Solid Edge part; units mm, degrees
sketch "Sketch1" plane through (0, 0, 0) normal (0, 0, 1) x (1, 0, 0)
  line L0 (20.5, -19.5) -> (28, -19.5)
  line L1 (28, -19.5) -> (28, -16.5)
  line L2 (28, -16.5) -> (24, -16.5)
  line L3 (24, -16.5) -> (24, 16.5)
  line L4 (24, 16.5) -> (28, 16.5)
  line L5 (28, 16.5) -> (28, 19.5)
  line L6 (28, 19.5) -> (20.5, 19.5)
  line L7 (20.5, -19.5) -> (20.5, 19.5)
revolve "RevolvedProtrusion1" add sketch "Sketch1" angle 180 about axis through (0, 54, 0) along (0, -1, 0)
sketch "Sketch2" plane through (0, 0, 0) normal (0, 0, 1) x (1, 0, 0)
  circle A0 centre (0, 0) radius 1
extrude "ExtrudedCutout_1" cut sketch "Sketch2" along normal mid plane 257.4558
sketch "Sketch3" plane through (0, 0, 0) normal (1, 0, 0) x (0, 1, 0)
  line L0 (-19.5, 0) -> (-19.5, 1.5)
  line L1 (-19.5, 1.5) -> (19.5, 1.5)
  line L2 (19.5, 1.5) -> (19.5, 0)
  line L3 (19.5, 0) -> (-19.5, 0)
extrude "ExtrudedCutout_2" cut sketch "Sketch3" along normal mid plane 153.986
Geometry: final body of the model. Coordinates: model frame, mm. A direction names the side the tool comes from. Give positions to 0.01 mm unless a question says otherwise; leave off trailing zeros. Order: outer loops, then holes, each group sorted by start corner. A loop starts at its lowest first (then second) coordinate and runs counter-clockwise, first axis right, second up. Notation, with made-up numbers: M 49,78 L 75,78 A11 cw 75,91 Z; hole C 58.5,-35.75 d1. An arc over 180 degrees is marked long. Answer as CSV lines item,"result". Start each with the question number.
1) Cut plane B-B (z = 25). Output: boundary loops of the cut face in (x, y).
2) Cut plane D-D (y = 0). Output: boundary loops of the cut face in (x, z).
3) First-contact query: P1, Ø5, axis at y = -1.5, z = 24, coming from the +X side; P2, Ø12, axis at y = 3.5, z = 25, coming from the +X side; P3, Ø3, axis at x = 5.5, y = 0.5, coming from the +Z side. Flat tips, straight axial feed; report the tip coordinate or a pass-through.
4) Set-up query: faces 1 (the flat face through (-2, 16.5, 25)), 2 (the cylindrical face through (-0.43, 4.606, 20.495)). Return all of +Z, -Z, +X, -X, +Y, -Y with unobstructed straight access to the full face (end or side cutting, diameter ignored); none if empty.
5) Line query: line 1 (Y direction, x = -2.5, z = 26); line 2 (Y direction, x = 0, z = 21.8); line 3 (X direction, y = 1.5, z = 10). Output: solid intervals per line, ascending. Write a range as from..to.
6) Mould query, pull axis Y, two halves, no side actions, for faces 3 (the flat face through (-2, -16.5, 25)), 4 (the flat face through (0, -19.5, 21)), 5 (the cylindrical face through (-0.595, -17.979, 27.994)), 6 (the cylindrical face through (-0.507, 3.898, 23.995)). Classes: +Y half, -Y half, draft (parallel to the pull), parting line (faces both ways), or undercut.
7) Cut plane A-A (x = 0). Output: boundary loops of the cut face in (y, z).
8) Cut plane C-C (z = 21.5). Output: boundary loops of the cut face in (x, y), then the cut area to 3 significant figures.
Findings below:
1,outline,"M -12.61,-19.5 L 12.61,-19.5 L 12.61,-16.5 L -12.61,-16.5 Z; M -12.61,16.5 L 12.61,16.5 L 12.61,19.5 L -12.61,19.5 Z"
2,outline,"M -23.95,1.5 L -20.45,1.5 A20.5 cw -1,20.48 L -1,23.98 A24 ccw Z; M 1,20.48 A20.5 cw 20.45,1.5 L 23.95,1.5 A24 ccw 1,23.98 Z"
3,P1,"stops at x = 10.67"
3,P2,"stops at x = 14.66"
3,P3,"stops at z = 23.66"
4,face 1,"+Z"
4,face 2,"-Z, +Y, -Y"
5,line 1,"y = -19.5..-16.5, 16.5..19.5"
5,line 2,"y = -19.5..-1, 1..19.5"
5,line 3,"x = -21.82..-17.9, 17.9..21.82"
6,face 3,"undercut"
6,face 4,"-Y half"
6,face 5,"draft"
6,face 6,"undercut"
7,outline,"M -19.5,20.5 L -1,20.5 L -1,24 L -16.5,24 L -16.5,28 L -19.5,28 Z; M 1,20.5 L 19.5,20.5 L 19.5,28 L 16.5,28 L 16.5,24 L 1,24 Z"
8,outline,"M -17.94,-19.5 L 17.94,-19.5 L 17.94,-16.5 L 10.67,-16.5 L 10.67,16.5 L 17.94,16.5 L 17.94,19.5 L -17.94,19.5 L -17.94,16.5 L -10.67,16.5 L -10.67,-16.5 L -17.94,-16.5 Z; hole C 0,0 d2"
8,area,"916 mm²"
